The listing builds one solid part. Answer for the finished solid, in the listing's coordinates (mm). Face numbers are marked on the shaded views. A direction names the side the tool comes from. Round coordinates to 2 decimals unless told otherwise and drop trailing zeros. Order: outer loops, then holes, each group sorted by start corner. A loop starts at its lowest first (then second) coordinate and runs counter-clockwise, first axis right, second up. Notation, with made-up numbers: (-39, 43.25) - (-4, 43.25) arc R21 ccw to (-4, 68.25) - close; hole circle Ø4 at (24, 5). An arc over 180 degrees is marked (long way). One line per item, written item: value. Start each with the question number.
1. Section C-C, the plane x = -102 is taken. Give the vertices of the cut face in (y, z), then the cut area to 3 significant figures.
2. Flat-ended cylindrical pins translate along their axes: P1, Ø1.5, axis at y = -23, z = -7.5, coming from the +X side; P2, Ø19, axis at x = -59.5, y = 1, coming from the -Z side; P3, Ø12, axis at x = -1, z = 20, coming from the +Y side; P4, Ø11, axis at x = -93, z = 26.5, coming from the -Y side. Find the tip coordinate at first contact, or state that the pin passes through.
3. Straight lines are drawn through the part: line 1 (Y direction, x = -135, z = 14); line 2 (Z direction, x = 7, y = 27.5); line 3 (Z direction, x = -22, y = 8). For each, find the intervals that lie inside material, in ascending order.
4. Section B-B, the plane z = 12 is taken. Give the vertices of the cut face in (x, y), then the cut area to 3 significant figures.
5. A tool of negligible diameter and unlimited length cuts with its end or side. For the marked faces 1, 2 and 3, from which of +Z, -Z, +X, -X, +Y, -Y can it reach the whole face along a straight path? Write none if from no direction.
6. For a pull along Z with two mould halves and no side action, classify the marked faces 4, 5, 6 and 7 as released by +Z, released by -Z, zero draft, split by the parting line, or undercut.
7. Section A-A, the plane y = 0 is taken. Give the vertices of the cut face in (x, z), then the cut area to 3 significant figures.
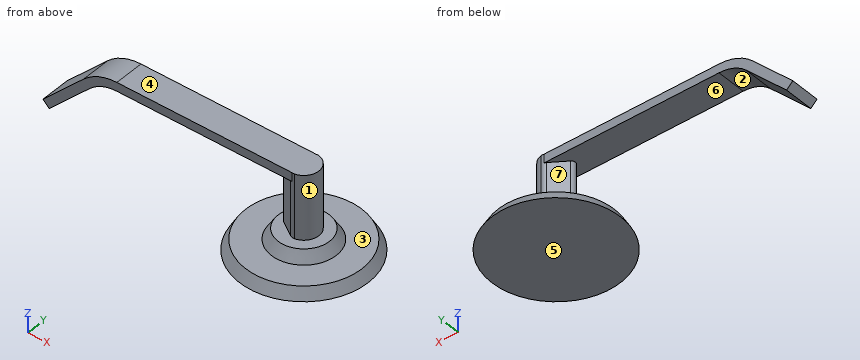
from build123d import *

# Parameters (mm, degrees)
BOSS_EXTRUDE1_DEPTH = 38.1
SKETCH3_W           = 5.185673946
SKETCH3_H           = 17.43749126


with BuildPart() as part:
    # Sketch1 → Revolve1 (revolve)
    with BuildSketch(Plane(origin=(0, 0, 0), x_dir=(1, 0, 0), z_dir=(0, 1, 0))):
        Polygon((0, 0), (0, 12.7), (38.1, 12.7), (34.433825791, 6.35), (19.193825791, 6.35), (15.24, 0), align=None)
    revolve(axis=Axis((0, 0, 0), (0, 0, -1)))

    # Sketch2 → Boss-Extrude1 (add)
    with BuildSketch(Plane.XY):
        with BuildLine():
            Line((-1.101928038, 8.164948968), (-10.28615812, 2.121872405))
            ThreePointArc((-10.28615812, 2.121872405), (-11.43, 0), (-10.28615812, -2.121872405))
            Line((-10.28615812, -2.121872405), (-1.101928038, -8.164948968))
            ThreePointArc((-1.101928038, -8.164948968), (0.26271934, -8.721632133), (1.736540998, -8.71874563))
            ThreePointArc((1.736540998, -8.71874563), (8.89, 0), (1.736540998, 8.71874563))
            ThreePointArc((1.736540998, 8.71874563), (0.26271934, 8.721632133), (-1.101928038, 8.164948968))
        make_face()
    extrude(amount=BOSS_EXTRUDE1_DEPTH)

    # Sweep1: sweep along a path in Sketch4
    with BuildLine(Plane(origin=(0, 0, 0), x_dir=(1, 0, 0), z_dir=(0, 1, 0))) as sweep1_path:
        Line((0, -35.507163027), (-103.778975516, -35.507163027))
        ThreePointArc((-103.778975516, -35.507163027), (-113.499134698, -33.573703153), (-121.739487758, -28.067675269))
        Line((-121.739487758, -28.067675269), (-145.730896424, -4.076266603))
    # Sketch3 → Sweep1 (sweep)
    with BuildSketch(Plane(origin=(0, 0, 0), x_dir=(0, 0, -1), z_dir=(1, 0, 0))):
        with Locations((-35.507163027, 0)):
            Rectangle(SKETCH3_W, SKETCH3_H)
    sweep(path=sweep1_path.line)


solid = part.part
Answer list:
1. outline: (-8.72, 32.91) - (8.72, 32.91) - (8.72, 38.1) - (-8.72, 38.1) - close
1. area: 90.4 mm²
2. P1: stops at x = 27.36
2. P2: stops at z = 32.91
2. P3: stops at y = 8.79
2. P4: passes through
3. line 1: y = -8.72 to 8.72
3. line 2: z = -12.7 to -6.35
3. line 3: z = -12.7 to -6.35, 32.91 to 38.1
4. outline: (-141.47, -8.72) - (-134.14, -8.72) - (-134.14, 8.72) - (-141.47, 8.72) - close; (-10.29, -2.12) - (-1.1, -8.16) arc R3.81 ccw to (1.74, -8.72) arc R8.89 ccw to (1.74, 8.72) arc R3.81 ccw to (-1.1, 8.16) - (-10.29, 2.12) arc R2.54 ccw to start
4. area: 368 mm²
5. face 1: +Z, +X
5. face 2: -Z, +Y, -Y
5. face 3: none
6. face 4: released by +Z
6. face 5: released by -Z
6. face 6: undercut
6. face 7: undercut
7. outline: (-147.56, 5.91) - (-143.9, 2.24) - (-119.91, 26.23) arc R22.81 cw to (-103.78, 32.91) - (-11.43, 32.91) - (-11.43, 0) - (-15.24, 0) - (-19.19, -6.35) - (-34.43, -6.35) - (-38.1, -12.7) - (38.1, -12.7) - (34.43, -6.35) - (19.19, -6.35) - (15.24, 0) - (8.89, 0) - (8.89, 38.1) - (-103.78, 38.1) arc R27.99 ccw to (-123.57, 29.9) - close
7. area: 2,210 mm²
